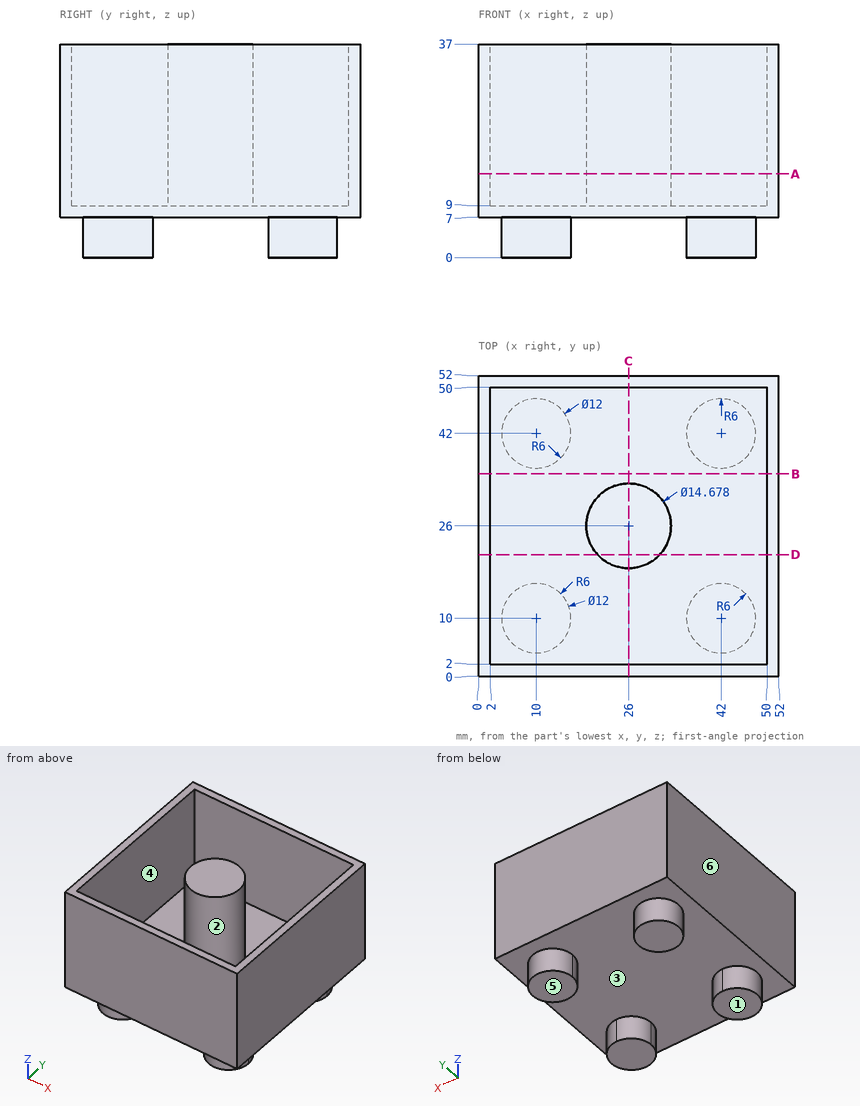
Part print with two shaded views. Sizes in mm from the minimum x, y, z corner. A direction names the side the tool comes from. Round coordinates to 2 decimals unless told otherwise and drop trailing zeros. Order: outer loops, then holes, each group sorted by start corner. A loop starts at its lowest first (then second) coordinate and runs counter-clockwise, first axis right, second up.
(1) Drill centre lines: line 1 (X direction, y = 37.5, z = 10.5); line 2 (Y direction, x = 32, z = 28.5). Where is each one in solid material? Low to high.
(2) Pin check, flat tips, straight feed: pin 1 (2 mm diameter, centred on x = 23.5, y = 30.5, fed in from -Z); pin 2 (6 mm diameter, centred on x = 40, y = 26, fed in from +Z). Stop position of each tip, or through.
(3) Band-saw the part on B-B (y = 35). List the corners of the cut face in (x, z), then the cut area to 3 significant figures.
(4) Pull direction X, two halves, no side cores. Call the marked faces 3, 4, 5 and 6: released by +X, released by -X, zero draft, split by the parting line, or undercut.
(5) Band-saw the part on A-A (z = 14.5). List the corners of the cut face in (x, y), then the cut area to 3 significant figures.
(6) 3-axis set-ups, long thin cutter, end or side, ignore diameter. For the marked faces 1 and 2: which of +Z, -Z, +X, -X, +Y, -Y reach the whole face in a straight line?
(7) Band-saw the part on D-D (y = 21). List the corners of the cut face in (x, z), then the cut area to 3 significant figures.
(8) Band-saw the part on C-C (x = 26). List the corners of the cut face in (y, z), then the cut area to 3 significant figures.
Verdict:
1. line 1: x = 0 to 2, 50 to 52
1. line 2: y = 0 to 2, 21.77 to 30.23, 50 to 52
2. pin 1: stops at z = 7
2. pin 2: stops at z = 9
3. outline: (0, 7) - (52, 7) - (52, 37) - (50, 37) - (50, 9) - (2, 9) - (2, 37) - (0, 37) - close
3. area: 216 mm2
4. face 3: undercut
4. face 4: undercut
4. face 5: zero draft
4. face 6: released by -X
5. outline: (0, 0) - (52, 0) - (52, 52) - (0, 52) - close; circle Ø14.68 at (26, 26); hole (2, 2) - (50, 2) - (50, 50) - (2, 50) - close
5. area: 569 mm2
6. face 1: -Z, +X, -X, +Y, -Y
6. face 2: +Z
7. outline: (0, 7) - (52, 7) - (52, 37) - (50, 37) - (50, 9) - (31.37, 9) - (31.37, 37) - (20.63, 37) - (20.63, 9) - (2, 9) - (2, 37) - (0, 37) - close
7. area: 517 mm2
8. outline: (0, 7) - (52, 7) - (52, 37) - (50, 37) - (50, 9) - (33.34, 9) - (33.34, 37) - (18.66, 37) - (18.66, 9) - (2, 9) - (2, 37) - (0, 37) - close
8. area: 627 mm2
